The listing builds one solid part. Answer for the finished solid, in the listing's coordinates (mm). Face numbers are marked on the shaded views. A direction names the side the tool comes from. Round coordinates to 2 decimals unless told otherwise and drop trailing zeros. Order: outer loops, then holes, each group sorted by start corner. A loop starts at its lowest first (then second) coordinate and runs counter-clockwise, first axis right, second up. Notation, with made-up numbers: (12.25, -10.5) - (28.25, -10.5) arc R23 cw to (28.25, 4.5) - close; hole circle Ø10 at (-38, -37.5). An arc over 180 degrees is marked (long way). Use CSV: the item, a comma, the result in double quotes. Start each with the question number.
Item 1: Straight lines are drawn through the part: line 1 along X through (y, z) = (2, 10); line 2 along Z through (x, y) = (8.5, 12); line 3 along X through (y, z) = (8, 16.5). For each, find the intervals that lie inside material, in ascending order. Write a range as [from, to].
Item 2: Find section D-D, the plane y = 13. Give the vertices of the cut face in (x, z).
Item 3: For the marked faces 1, 2 and 3, determine the directions among +Z, -Z, +X, -X, +Y, -Y from which every point of the face is accessible in a straight line to the end or side of a thin tool.
Item 4: Flat-ended cylindrical pins translate along their axes: P1, Ø2.5, axis at x = 28.5, z = 3, coming from the +Y side; P2, Ø7, axis at x = 7, y = 8, coming from the +Z side; P3, Ø1.2, axis at x = -29.5, y = 2, coming from the +Z side; P4, Ø12, axis at x = 9, z = -11, coming from the -Y side. Find the tip coordinate at first contact, or state that the pin passes through.
Item 5: Find section B-B, the plane y = 1.25. Give the vertices of the cut face in (x, z), plus the area to 3 significant figures.
Item 6: Find section A-A, the plane x = 19.25. Give the vertices of the cut face in (y, z).
Item 7: Find section C-C, the plane x = -19. Give the vertices of the cut face in (y, z).
Item 8: Determine the mould class of the marked faces 4, 5, 6 and 7 for opening direction X: +X half, -X half, draft (parallel to the pull), parting line (faces both ways), or undercut.
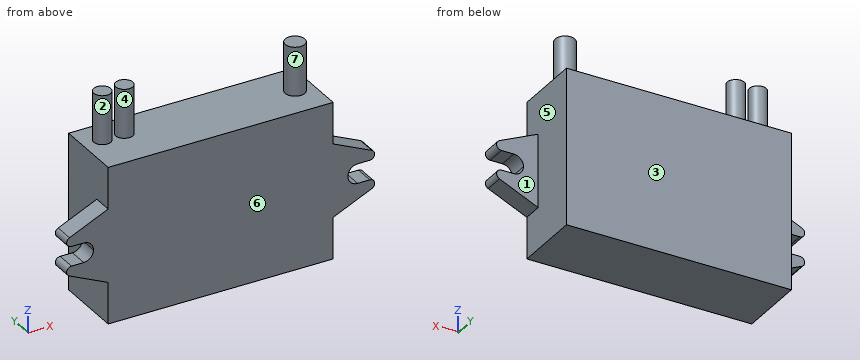
```python
from build123d import *

# Parameters (mm, degrees)
SKETCH1_W            = 46
SKETCH1_H            = 32
BOSS_EXTRUDE1_DEPTH  = 14
BOSS_EXTRUDE2_DEPTH  = 4
MIRROR2_COPY_1_DEPTH = 4
SKETCH3_R            = 1.75
SKETCH3_R_2          = 2
BOSS_EXTRUDE3_DEPTH  = 10


with BuildPart() as part:
    # Sketch1 → Boss-Extrude1 (new body)
    with BuildSketch(Plane(origin=(0, 0, 0), x_dir=(1, 0, 0), z_dir=(0, 1, 0))):
        Rectangle(SKETCH1_W, SKETCH1_H)
    extrude(amount=BOSS_EXTRUDE1_DEPTH)

    # Sketch2 → Boss-Extrude2 (add)
    with BuildSketch(Plane.XZ):
        with BuildLine():
            Line((-28, 2), (-30.5, 2))
            ThreePointArc((-30.5, 2), (-31.477418408, 2.788686832), (-30.913082761, 3.91069349))
            Line((-30.913082761, 3.91069349), (-23, 7.5))
            Line((-23, 7.5), (-23, 0))
            Line((-23, 0), (-26, 0))
            ThreePointArc((-26, 0), (-26.585786438, 1.414213562), (-28, 2))
        make_face()
    boss_extrude2 = extrude(amount=-BOSS_EXTRUDE2_DEPTH)

    # Mirror1: Boss-Extrude2 across plane
    add(boss_extrude2.mirror(Plane.XY))

    # Mirror2: Boss-Extrude2 across plane
    add(boss_extrude2.mirror(Plane(origin=(0, 0, 0), x_dir=(0, 0, 1), z_dir=(1, 0, 0))))

    # Mirror2 copy 1 sketch → Mirror2 copy 1 (add)
    with BuildSketch(Plane(origin=(0, 0, 0), x_dir=(-1, 0, 0), z_dir=(0, -1, 0))):
        with BuildLine():
            Line((-28, 2), (-30.5, 2))
            ThreePointArc((-30.5, 2), (-31.477418408, 2.788686832), (-30.913082761, 3.91069349))
            Line((-30.913082761, 3.91069349), (-23, 7.5))
            Line((-23, 7.5), (-23, 0))
            Line((-23, 0), (-26, 0))
            ThreePointArc((-26, 0), (-26.585786438, 1.414213562), (-28, 2))
        make_face()
    extrude(amount=-MIRROR2_COPY_1_DEPTH)

    # Sketch3 → Boss-Extrude3 (add)
    with BuildSketch(Plane.XY.offset(16)):
        with Locations((-19, 9)):
            Circle(SKETCH3_R)
        with Locations((-14.5, 9)):
            Circle(SKETCH3_R)
        with Locations((19.25, 7)):
            Circle(SKETCH3_R_2)
    extrude(amount=BOSS_EXTRUDE3_DEPTH)


solid = part.part
```
Worked out:
1,line 1,"x = [-23, 23]"
1,line 2,"z = [-16, 16]"
1,line 3,"x = [-20.44, -17.56], [-15.94, -13.06], [17.52, 20.98]"
2,outline,"(-23, -16) - (23, -16) - (23, 16) - (-23, 16) - close"
3,face 1,"+Z, -Z, +X, +Y"
3,face 2,"+Z"
3,face 3,"+Z, -Z, +X, -X, +Y"
4,P1,"stops at y = 4"
4,P2,"stops at z = 16"
4,P3,"stops at z = 4.82"
4,P4,"stops at y = 0"
5,outline,"(-30.91, -3.91) - (-23, -7.5) - (-23, -16) - (23, -16) - (23, -7.5) - (30.91, -3.91) arc R1 ccw to (30.5, -2) - (28, -2) arc R2 cw to (28, 2) - (30.5, 2) arc R1 ccw to (30.91, 3.91) - (23, 7.5) - (23, 16) - (-23, 16) - (-23, 7.5) - (-30.91, 3.91) arc R1 ccw to (-30.5, 2) - (-28, 2) arc R2 cw to (-28, -2) - (-30.5, -2) arc R1 ccw to start"
5,area,"1,620 mm²"
6,outline,"(0, -16) - (14, -16) - (14, 16) - (9, 16) - (9, 26) - (5, 26) - (5, 16) - (0, 16) - close"
7,outline,"(0, -16) - (14, -16) - (14, 16) - (10.75, 16) - (10.75, 26) - (7.25, 26) - (7.25, 16) - (0, 16) - close"
8,face 4,"undercut"
8,face 5,"+X half"
8,face 6,"draft"
8,face 7,"undercut"
